Autodesk Inventor part; units mm, degrees
ref_plane "YZ Plane" through (0, 0, 0) normal (1, 0, 0) x (0, 1, 0)
ref_plane "XZ Plane" through (0, 0, 0) normal (0, 1, 0) x (-1, 0, 0)
ref_plane "XY Plane" through (0, 0, 0) normal (0, 0, 1) x (1, 0, 0)
sketch "Sketch1" plane through (0, 0, 0) normal (0, 0, 1) x (1, 0, 0)
  line L0 (-60, -17.5) -> (0, -17.5)
  line L1 (60, -17.5) -> (60, 17.5) construction
  line L2 (60, 17.5) -> (55, 17.5) construction
  line L3 (-60, 17.5) -> (-60, -17.5)
  line L4 (-60, -17.5) -> (60, 17.5) construction
  line L5 (60, -17.5) -> (-60, 17.5) construction
  line L6 (-55, -12.5) -> (0, -12.5)
  line L7 (55, -12.5) -> (55, 12.5) construction
  line L8 (55, 12.5) -> (-55, 12.5) construction
  line L9 (-55, 12.5) -> (-55, -12.5)
  line L10 (-55, 12.5) -> (-55, 17.5)
  line L11 (55, 12.5) -> (55, 17.5) construction
  line L12 (-55, 17.5) -> (-60, 17.5)
  line L13 (55, 17.5) -> (-55, 17.5) construction
  line L14 (0, -17.5) -> (0, 17.5)
  line L15 (0, -12.5) -> (55, -12.5) construction
  line L16 (0, -17.5) -> (60, -17.5) construction
  line L17 (0, -12.5) -> (0, -17.5)
  line L18 (0, 17.5) -> (-55, 17.5)
  point P0 (0, 0)
  dimension "d0" = 120
  dimension "d1" = 35
  dimension "d2" = 5
  dimension "d3" = 5
  dimension "d4" = 5
  dimension "d5" = 30
revolve "Revolution1" add sketch "Sketch1" angle 180 about axis through (0, -17.5, 0) along (0, 1, 0) contours L3 L12 L10 L9 L6 L14 L0
sketch "Sketch2" plane through (60, -17.5, 0) normal (0, 0, -1) x (-1, 0, 0)
  line L0 (0, 35) -> (0, 0)
  line L1 (0, 0) -> (60, 0) construction
  line L2 (120, 0) -> (0, 0)
  line L3 (60, 0) -> (60, 35) construction
  line L4 (60, 0) -> (60, 5) construction
  line L5 (60, 5) -> (35, 5)
  line L6 (35, 5) -> (35, 35)
  line L7 (35, 35) -> (30, 35)
  line L8 (30, 35) -> (30, 0)
  line L9 (60, 5) -> (85, 5)
  line L10 (85, 5) -> (85, 35)
  line L11 (85, 35) -> (90, 35)
  line L12 (90, 35) -> (90, 0)
  point P0 (60, 17.5)
  dimension "d7" = 60
  dimension "d8" = 35
  dimension "d9" = 5
  dimension "d10" = 25
  dimension "d11" = 30
  dimension "d12" = 5
extrude "Extrusion1" add sketch "Sketch2" against normal blind 150
sketch "Sketch3" plane through (60, -17.5, 0) normal (0, 0, -1) x (-1, 0, 0)
  line L0 (35, 35) -> (35, 5)
  line L1 (85, 5) -> (35, 5)
  line L2 (85, 5) -> (85, 35)
  line L3 (85, 35) -> (35, 35)
  point P0 (60, 17.5)
extrude "Extrusion2" cut sketch "Sketch3" against normal through all
revolve "Revolution2" cut sketch "Sketch1" angle 360 about axis through (0, -17.5, 0) along (0, 1, 0) contours L6 L9 L10 L18 L14
properties part number "select end track"
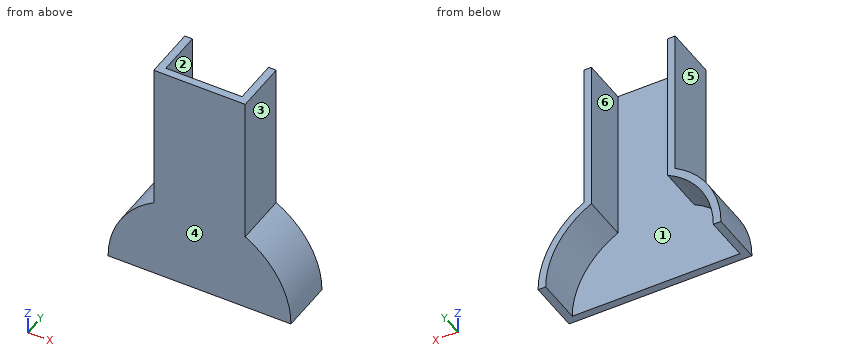
Here's how the part is built. I have some questions about the finished solid (model axes, mm). Face numbers are marked on the shaded views. A direction names the side the tool comes from. Give positions to 0.01 mm unless a question says otherwise; leave off trailing zeros. Write each loop counter-clockwise with the first axis right and the second up, starting at its lowest first coordinate (ties: lowest second). Pieces come first, ordered by that corner, then holes.
(1) On a 3-axis mill with a long thin cutter (end or side, diameter ignored), from which of +Z, -Z, +X, -X, +Y, -Y can I reach the whole of each face in a straight line? I mean the marked faces 1, 2 and 3. Say none if no direction works.
Output values:
face 1: -Z, +Y
face 2: +Z, -Z, +Y
face 3: +Z, +X, +Y, -Y
(2) Imagine slicing it at D-D, the plane z = 33. Write out the boundary of the cut face in (x, y).
Output values:
outline: (-50.11, -17.5) - (50.11, -17.5) - (50.11, 17.5) - (44, 17.5) - (44, -12.5) - (-44, -12.5) - (-44, 17.5) - (-50.11, 17.5) - close
(3) Thinking about a two-plate mould opening in X: for the marked faces 4, 5 and 6, which applies, pulls with the +X half, pulls with the -X half, needs draft (parallel to the pull), parting line crosses it, or undercut?
Output values:
face 4: needs draft
face 5: pulls with the -X half
face 6: undercut
(4) Will these pins go through, and if not, where does the flat tip stop? pin 1 (4 mm diameter, centred on x = -27, z = 18, fed in from +Y); pin 2 (6 mm diameter, centred on y = -7.5, z = 39, fed in from -X); pin 3 (17.5 mm diameter, centred on y = 0.5, z = 87.5, fed in from +X).
Output values:
pin 1: stops at y = -12.5
pin 2: stops at x = -48
pin 3: stops at x = 30
(5) Imagine slicing it at A-A, the plane y = 14. Write out the boundary of the cut face in (x, z).
Output values:
outline: (-60, 0) - (-55, 0) arc R55 cw to (-25, 48.99) - (-25, 150) - (-30, 150) - (-30, 51.96) arc R60 ccw to start; (25, 48.99) arc R55 cw to (55, 0) - (60, 0) arc R60 ccw to (30, 51.96) - (30, 150) - (25, 150) - close
(6) Imagine slicing it at B-B, the plane z = 120.5. Write out the boundary of the cut face in (x, y).
Output values:
outline: (-30, -17.5) - (30, -17.5) - (30, 17.5) - (25, 17.5) - (25, -12.5) - (-25, -12.5) - (-25, 17.5) - (-30, 17.5) - close
(7) Imagine slicing it at C-C, the plane x = 50.5. Write out the boundary of the cut face in (y, z), and give its area (3 significant figures).
Output values:
outline: (-17.5, 0) - (-12.5, 0) - (-12.5, 21.79) - (17.5, 21.79) - (17.5, 32.4) - (-17.5, 32.4) - close
area: 480 mm2
(8) If I drill on L1, parallel to X at y = 3, z = 108; L2, parallel to Y at x = 20, z = 78; L3, parallel to X at y = 5, z = 51, over which ranges is the centre line in solid material (lowest first)?
Output values:
L1: x = -30 to -25, 25 to 30
L2: y = -17.5 to -12.5
L3: x = -31.61 to -25, 25 to 31.61
